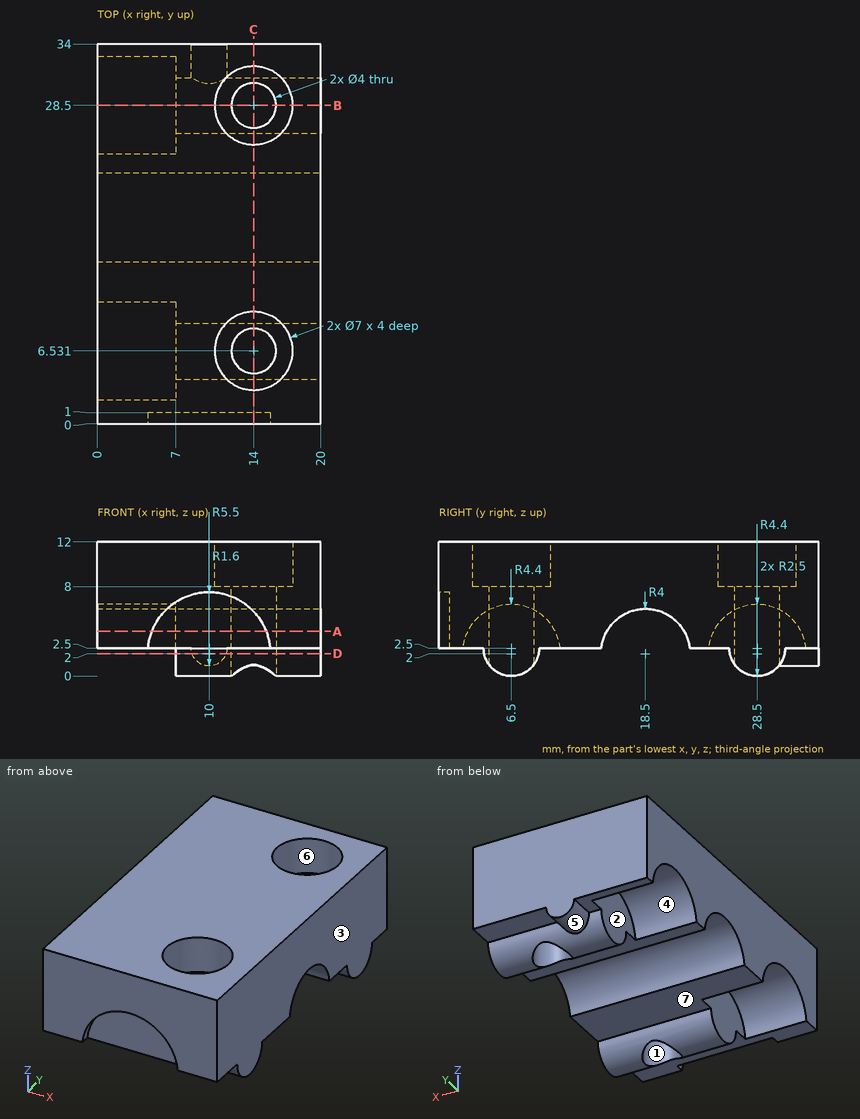
Verification items for this drawing (mm, ordinates from the low corner). A direction names the side the tool comes from. Coordinates: 2 decimals unless noted, no trailing zeros. Loops run counter-clockwise (first coordinate to the right, second up) from the corner with the lowest first, then second, coordinate; pieces in that order, holes last. Notation, with made-up numbers: (-40, 62.25) - (-12, 62.25) arc R24 cw to (-12, 82.25) - close; hole circle Ø11 at (65.5, -32.75). An arc over 180 degrees is marked (long way). Answer as a JSON object with one key per item and string values.
(1) Go/stop test with flat-tipped pins: pin 1 Ø2.5 at (x, y) = (17.5, 32.5) entering from -Z; pin 2 Ø1.5 at (x, z) = (8.5, 4.5) entering from -Y; pin 3 Ø3.5 at (x, y) = (13, 7) entering from +Z. Record where each tip stops, or that it passes through.
Response:
{"pin 1": "stops at z = 2.5", "pin 2": "stops at y = 1", "pin 3": "stops at z = 8"}
(2) Cross-section at A-A, the plane z = 4. Record the boundary of the cut face in (x, y), then the cut area to 3 significant figures.
Response:
{"outline": "(0, 0) - (4.88, 0) - (4.88, 1) - (15.12, 1) - (15.12, 0) - (20, 0) - (20, 15.04) - (0, 15.04) - (0, 10.42) - (7, 10.42) - (7, 2.58) - (0, 2.58) - close; (0, 21.96) - (20, 21.96) - (20, 34) - (0, 34) - (0, 32.42) - (7, 32.42) - (7, 24.58) - (0, 24.58) - close; hole circle Ø4 at (14, 6.53); hole circle Ø4 at (14, 28.5)", "area": "396 mm²"}
(3) Cross-section at D-D, the plane z = 2. Record the boundary of the cut face in (x, y).
Response:
{"outline": "(7, 4.05) - (20, 4.05) - (20, 8.95) - (7, 8.95) - close; (7, 26.05) - (20, 26.05) - (20, 30.95) - (11.52, 30.95) - (11.52, 34) - (8.48, 34) - (8.48, 30.95) - (7, 30.95) - close; hole circle Ø4 at (14, 6.53); hole circle Ø4 at (14, 28.5)"}
(4) Cross-section at C-C, the plane x = 14. Record the boundary of the cut face in (y, z) (1 decimal), then the cut area to 3 significant figures.
Response:
{"outline": "(0, 5.8) - (1, 5.8) - (1, 2.5) - (4, 2.5) arc R2.5 ccw to (4.5, 1) - (4.5, 8) - (3, 8) - (3, 12) - (0, 12) - close; (8.5, 1) arc R2.5 ccw to (9, 2.5) - (14.5, 2.5) arc R4 cw to (22.5, 2.5) - (26, 2.5) arc R2.5 ccw to (26.5, 1) - (26.5, 8) - (25, 8) - (25, 12) - (10, 12) - (10, 8) - (8.5, 8) - close; (30.5, 1) arc R2.5 ccw to (31, 2.5) - (34, 2.5) - (34, 12) - (32, 12) - (32, 8) - (30.5, 8) - close", "area": "201 mm²"}
(5) Mould release check, pull along X, two halves, no side actions. Record for the marked faces 1, 2, 3 and 4: pulls with the +X half, pulls with the -X half, needs draft (parallel to the pull), parting line crosses it, or undercut.
Response:
{"face 1": "undercut", "face 2": "pulls with the -X half", "face 3": "pulls with the +X half", "face 4": "needs draft"}
(6) Access from +Z, -Z, +X, -X, +Y, -Y to the whole of each face (thin tool, end or side, straight path). Record for the marked faces 5, 6 and 7.
Response:
{"face 5": "-Z, +Y", "face 6": "+Z", "face 7": "-Z, +X, -X"}
(7) Cross-section at B-B, the plane y = 28.5. Record the boundary of the cut face in (x, z).
Response:
{"outline": "(0, 6.4) - (7, 6.4) - (7, 0) - (12, 0) - (12, 8) - (10.5, 8) - (10.5, 12) - (0, 12) - close; (16, 0) - (20, 0) - (20, 12) - (17.5, 12) - (17.5, 8) - (16, 8) - close"}
(8) Scan lines: line 1 along Y through (x, z) = (14, 9); line 2 along X through (y, z) = (28.5, 6.25); line 3 along Z through (x, y) = (13.5, 2). Record each from-to range of solid material in increasing order.
Response:
{"line 1": "y = 0 to 3.03, 10.03 to 25, 32 to 34", "line 2": "x = 7 to 12, 16 to 20", "line 3": "z = 2.5 to 12"}
